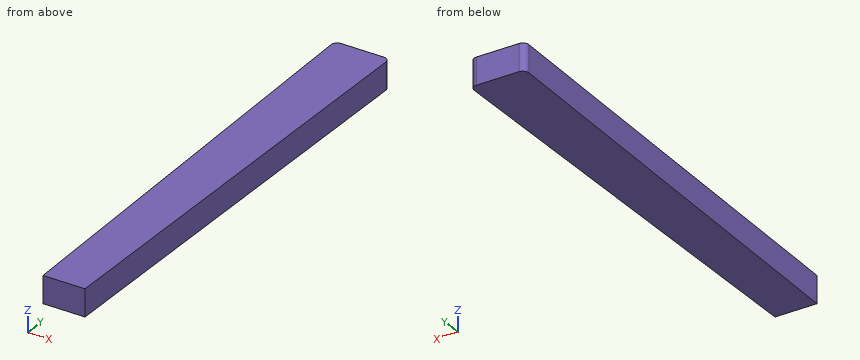
from build123d import *

# Parameters (mm, degrees)
F2_W = 42.8625
F2_H = 27.94
F0_W = 56.1086
F0_H = 27.94
F4_R = 6.35


with BuildPart() as f3:
    # F2 (on offset) → F3 section 0
    with BuildSketch(Plane.XZ.offset(476.25)):
        Rectangle(F2_W, F2_H)
    # F0 (on Front) → F3 section 1
    with BuildSketch(Plane.XZ):
        Rectangle(F0_W, F0_H)
    loft()

    # F4
    f4_edges = [f3.edges().sort_by_distance(p)[0] for p in [
        (-28.0543, 0, 0),
        (28.0543, 0, 0),
    ]]
    fillet(f4_edges, radius=F4_R)


solid = f3.part
Could you check a few things on this model? Use its own coordinates, in mm. Coordinates: 2 decimals unless noted, no trailing zeros. Write each loop counter-clockwise with the first axis right and the second up, starting at its lowest first coordinate (ties: lowest second). Pieces come first, ordered by that corner, then holes. Notation, with made-up numbers: (-31, 79) - (-6, 79) arc R22 cw to (-6, 86) - close; hole circle Ø3 at (83.25, 63.25). An arc over 180 degrees is marked (long way). Write item = value, one per line.
1) Suppose I cut it at A-A on z = 9.25. Please give me the cut outline in (x, y), plus the area to 3 significant figures.
Result set:
outline = (-27.96, -6.44) - (-21.43, -476.25) - (21.43, -476.25) - (27.96, -6.44) arc R6.35 ccw to (21.62, 0) - (-21.62, 0) arc R6.35 ccw to start
area = 23,500 mm2
2) Will these pins go through, and if not, where does the flat tip stop? pin 1 Ø1 at (y, z) = (-92, 3) entering from -X; pin 2 Ø10 at (y, z) = (-339, -2) entering from -X; pin 3 Ø12 at (y, z) = (-356, -3.5) entering from +X.
Result set:
pin_1 = -26.78
pin_2 = -23.41
pin_3 = 23.19
3) Please list where these lines run through material, in increasing order: line 1 (X direction, y = -425, z = -2.25); line 2 (X direction, y = -236, z = -3). Write a range as [from, to].
Result set:
line_1 = [-22.14, 22.14]
line_2 = [-24.77, 24.77]
